Geometry check sheet. Reference: the model listing, model coordinates, mm. Face numbers are marked on the shaded views. A direction names the side the tool comes from. Give positions to 0.01 mm unless a question says otherwise; leave off trailing zeros. Loops run counter-clockwise (first coordinate to the right, second up) from the corner with the lowest first, then second, coordinate; pieces in that order, holes last. Notation, with made-up numbers: (47, 88.25) - (82, 88.25) arc R25 cw to (82, 119.25) - close; hole circle Ø7 at (-31.5, -21.75). An arc over 180 degrees is marked (long way). Use a Markdown table: item, result. Add a question column.
1. Cross-section at C-C on x = -13. Enter the section's corners in (y, z).
2. Cross-section at B-B on y = -13. Enter the section's corners in (x, z), and give its area (3 significant figures).
3. Set-up check for the marked faces 1, 2 and 3: record each of +Z, -Z, +X, -X, +Y, -Y from which the full face is reachable in a straight line by a thin tool's end or side.
4. Depth check by flat-ended pin: P1, Ø11.5, axis at x = 6.5, y = 70.5, coming from the +Z side; P2, Ø12, axis at x = -2.5, z = 27.5, coming from the -Y side; P3, Ø19, axis at x = 5.5, y = -5, coming from the +Z side; P4, Ø5, axis at x = 3, z = 11.5, coming from the +Y side. Enter the tip coordinate at first touch or a pass-through.
5. Cross-section at D-D on z = 29.5. Enter the section's corners in (x, y), and give its area (3 significant figures).
6. Cross-section at A-A on z = 13.5. Enter the section's corners in (x, y).
7. Material ranges on L1, parallel to Y at x = 0, z = -3.5; L2, parallel to Y at x = 0, z = 18.05; L3, parallel to Y at x = 8, z = 7.5, recorded low to high.
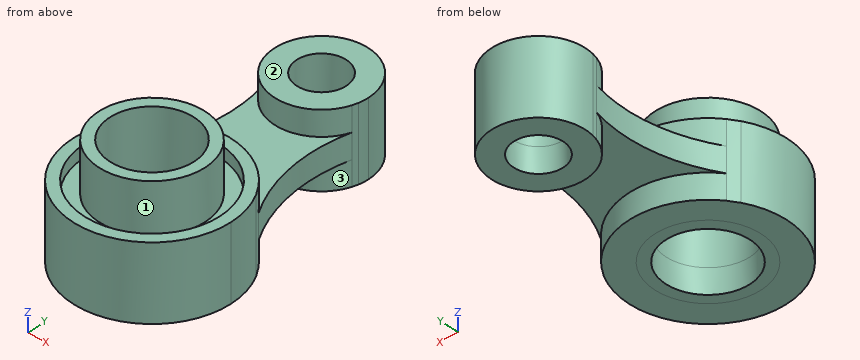
from build123d import *

# Parameters (mm, degrees)
BOSS_EXTRUDE6_DEPTH       = 10
SKETCH1_11_R              = 27.5
BOSS_EXTRUDE10_DEPTH      = 20
BOSS_EXTRUDE10_DEPTH_BACK = 10
SKETCH1_12_R              = 10
BOSS_EXTRUDE11_DEPTH      = 20
BOSS_EXTRUDE11_DEPTH_BACK = 10
SKETCH1_13_R              = 27.5
SKETCH1_13_R_2            = 21.5
BOSS_EXTRUDE12_DEPTH      = 15
BOSS_EXTRUDE12_DEPTH_BACK = 10
SKETCH1_14_R              = 21.5
SKETCH1_14_R_2            = 17
BOSS_EXTRUDE13_DEPTH      = 35
BOSS_EXTRUDE13_DEPTH_BACK = 10


with BuildPart() as part:
    # Sketch1 → Boss-Extrude6 (new body)
    with BuildSketch(Plane.XY):
        with BuildLine():
            ThreePointArc((-25.420986444, 19.436394938), (0, 32), (25.420986444, 19.436394938))
            ThreePointArc((25.420986444, 19.436394938), (16.698881669, 43.372332346), (17.965602149, 68.816381365))
            ThreePointArc((17.965602149, 68.816381365), (0, 56), (-17.965602149, 68.816381365))
            ThreePointArc((-17.965602149, 68.816381365), (-16.698881669, 43.372332346), (-25.420986444, 19.436394938))
        make_face()
    extrude(amount=BOSS_EXTRUDE6_DEPTH)

    # Sketch1_11 → Boss-Extrude10 (add, two sides)
    with BuildSketch(Plane.XY) as boss_extrude10_sk:
        with BuildLine():
            ThreePointArc((-27.861197674, 15.740192635), (-8.137618645, -30.948007412), (32, 0))
            ThreePointArc((32, 0), (30.948007412, 8.137618645), (27.861197674, 15.740192635))
            ThreePointArc((27.861197674, 15.740192635), (26.609230485, 17.567258961), (25.420986444, 19.436394938))
            ThreePointArc((25.420986444, 19.436394938), (0, 32), (-25.420986444, 19.436394938))
            ThreePointArc((-25.420986444, 19.436394938), (-26.609230485, 17.567258961), (-27.861197674, 15.740192635))
        make_face()
        Circle(SKETCH1_11_R, mode=Mode.SUBTRACT)
    extrude(amount=BOSS_EXTRUDE10_DEPTH)
    extrude(boss_extrude10_sk.sketch, amount=-BOSS_EXTRUDE10_DEPTH_BACK)

    # Sketch1_12 → Boss-Extrude11 (add, two sides)
    with BuildSketch(Plane.XY) as boss_extrude11_sk:
        with BuildLine():
            ThreePointArc((-17.965602149, 68.816381365), (0, 56), (17.965602149, 68.816381365))
            ThreePointArc((17.965602149, 68.816381365), (18.273648583, 69.980415685), (18.603456766, 71.138472275))
            ThreePointArc((18.603456766, 71.138472275), (18.900604204, 73.059082504), (19, 75))
            ThreePointArc((19, 75), (-1.940917496, 93.900604204), (-18.603456766, 71.138472275))
            ThreePointArc((-18.603456766, 71.138472275), (-18.273648583, 69.980415685), (-17.965602149, 68.816381365))
        make_face()
        with Locations((0, 75)):
            Circle(SKETCH1_12_R, mode=Mode.SUBTRACT)
    extrude(amount=BOSS_EXTRUDE11_DEPTH)
    extrude(boss_extrude11_sk.sketch, amount=-BOSS_EXTRUDE11_DEPTH_BACK)

    # Sketch1_13 → Boss-Extrude12 (add, two sides)
    with BuildSketch(Plane.XY) as boss_extrude12_sk:
        Circle(SKETCH1_13_R)
        Circle(SKETCH1_13_R_2, mode=Mode.SUBTRACT)
    extrude(amount=BOSS_EXTRUDE12_DEPTH)
    extrude(boss_extrude12_sk.sketch, amount=-BOSS_EXTRUDE12_DEPTH_BACK)

    # Sketch1_14 → Boss-Extrude13 (add, two sides)
    with BuildSketch(Plane.XY) as boss_extrude13_sk:
        Circle(SKETCH1_14_R)
        Circle(SKETCH1_14_R_2, mode=Mode.SUBTRACT)
    extrude(amount=BOSS_EXTRUDE13_DEPTH)
    extrude(boss_extrude13_sk.sketch, amount=-BOSS_EXTRUDE13_DEPTH_BACK)


solid = part.part
Values found:
| question | item | result |
|---|---|---|
| 1 | outline | (-29.24, -10) - (-10.95, -10) - (-10.95, 35) - (-17.12, 35) - (-17.12, 15) - (-24.23, 15) - (-24.23, 20) - (-29.24, 20) - close; (10.95, -10) - (29.24, -10) - (29.24, 0) - (61.14, 0) - (61.14, -10) - (88.86, -10) - (88.86, 20) - (61.14, 20) - (61.14, 10) - (29.24, 10) - (29.24, 20) - (24.23, 20) - (24.23, 15) - (17.12, 15) - (17.12, 35) - (10.95, 35) - close |
| 2 | outline | (-29.24, -10) - (-10.95, -10) - (-10.95, 35) - (-17.12, 35) - (-17.12, 15) - (-24.23, 15) - (-24.23, 20) - (-29.24, 20) - close; (10.95, -10) - (29.24, -10) - (29.24, 20) - (24.23, 20) - (24.23, 15) - (17.12, 15) - (17.12, 35) - (10.95, 35) - close |
| 2 | area | 1,210 mm2 |
| 3 | face 1 | +Z |
| 3 | face 2 | +Z, +X, -X, +Y |
| 3 | face 3 | -Z |
| 4 | P1 | stops at z = 20 |
| 4 | P2 | stops at y = -21.5 |
| 4 | P3 | passes through |
| 4 | P4 | stops at y = 93.99 |
| 5 | outline | circle Ø43 at (0, 0); hole circle Ø34 at (0, 0) |
| 5 | area | 544 mm2 |
| 6 | outline | (-27.86, 15.74) arc R32 ccw (long way) to (27.86, 15.74) arc R64.24 cw to (25.42, 19.44) arc R32 ccw to (-25.42, 19.44) arc R64.24 cw to start; (-18.6, 71.14) arc R64.24 cw to (-17.97, 68.82) arc R19 ccw to (17.97, 68.82) arc R64.24 cw to (18.6, 71.14) arc R19 ccw (long way) to start; hole circle Ø34 at (0, 0); hole circle Ø20 at (0, 75) |
| 7 | L1 | y = -32 to -17, 17 to 32, 56 to 65, 85 to 94 |
| 7 | L2 | y = -32 to -27.5, -21.5 to -17, 17 to 21.5, 27.5 to 32, 56 to 65, 85 to 94 |
| 7 | L3 | y = -30.98 to -15, 15 to 69, 81 to 92.23 |
